The drawing under review shows one solid part. Ordinate dimensions are in mm from its lowest x, y, z. A direction names the side the tool comes from. Coordinates: 2 decimals unless noted, no trailing zeros. Write each loop counter-clockwise with the first axis right and the second up, starting at its lowest first coordinate (ties: lowest second). Pieces come first, ordered by that corner, then holes.
1) Add section C-C, the plane x = 12. State the section outline as (y, z) points.
2) Add section D-D, the plane y = 4. State the section outline as (x, z) points.
3) Machinability: for the marked faces 5 and 6, which of the approach directions +Z, -Z, +X, -X, +Y, -Y give a long, thin tool a straight path to every point of the face, cutting with its end or side? Answer none if there is none.
4) Mouldability with a two-part tool opening along X and no side actions: class the marked faces 1, 2, 3 and 4 as released by +X, released by -X, zero draft, split by the parting line, or undercut.
5) For P1, Ø2, axis at x = 59.5, z = 1, coming from the +Y side; P2, Ø2.5, axis at y = 13, z = 5.5, coming from the -X side; P3, Ø1.5, axis at x = 8, z = 6, coming from the +Y side, all flat-tipped, find the tip position at first contact; note any pin that passes through.
6) For line 1 (Z direction, x = 12, y = 4); line 2 (Y direction, x = 29.5, z = 1.25); line 3 (X direction, y = 15, z = 5), list the stretches that pass through material, from the lowest coordinate up.
7) Add section A-A, the plane y = 8.75. State the section outline as (x, z) points.
8) Add section B-B, the plane z = 4. State the section outline as (x, y) points.
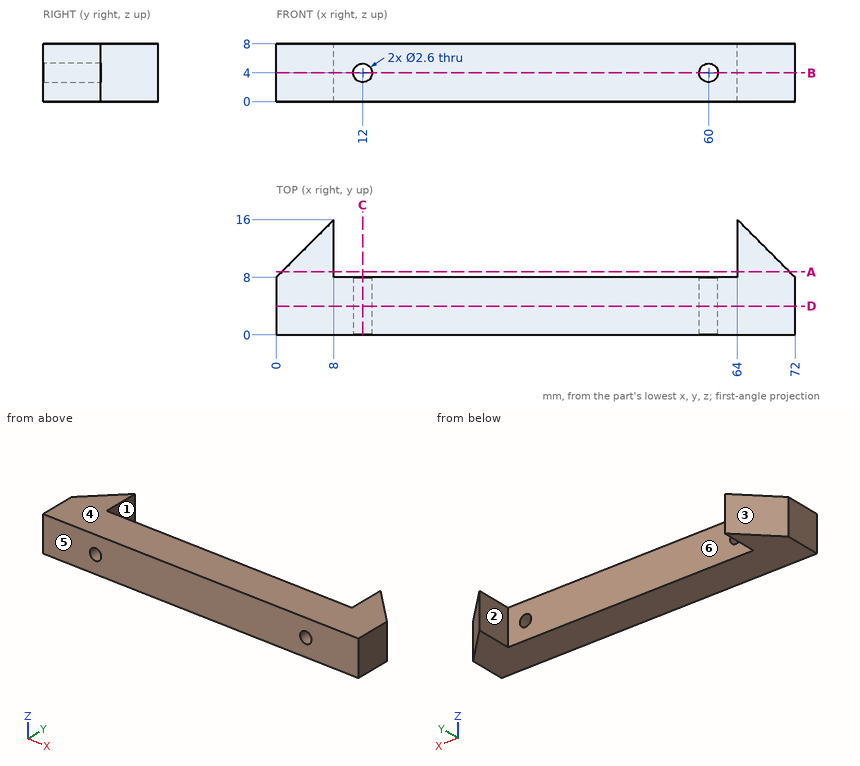
Geometry results:
1. outline: (0, 0) - (8, 0) - (8, 2.7) - (0, 2.7) - close; (0, 5.3) - (8, 5.3) - (8, 8) - (0, 8) - close
2. outline: (0, 0) - (72, 0) - (72, 8) - (0, 8) - close; hole circle Ø2.6 at (12, 4); hole circle Ø2.6 at (60, 4)
3. face 5: +Z, -Z, +X, -X, -Y
3. face 6: +Z, -Z, +Y
4. face 1: undercut
4. face 2: undercut
4. face 3: released by -X
4. face 4: zero draft
5. P1: stops at y = 8
5. P2: stops at x = 3.75
5. P3: stops at y = 16
6. line 1: z = 0 to 2.7, 5.3 to 8
6. line 2: y = 0 to 8
6. line 3: x = 7 to 8, 64 to 65
7. outline: (0.75, 0) - (8, 0) - (8, 8) - (0.75, 8) - close; (64, 0) - (71.25, 0) - (71.25, 8) - (64, 8) - close
8. outline: (0, 0) - (10.7, 0) - (10.7, 8) - (8, 8) - (8, 16) - (0, 8) - close; (13.3, 0) - (58.7, 0) - (58.7, 8) - (13.3, 8) - close; (61.3, 0) - (72, 0) - (72, 8) - (64, 16) - (64, 8) - (61.3, 8) - close
